Work out the finished part from the listing and answer in its coordinate system (mm). A direction names the side the tool comes from. Coordinates: 2 decimals unless noted, no trailing zeros. Order: outer loops, then holes, each group sorted by start corner. A loop starts at its lowest first (then second) coordinate and runs counter-clockwise, first axis right, second up. Notation, with made-up numbers: M 62.25,71 L 102.25,71 A21 cw 102.25,110 Z; hole C -25,3.5 d7. An arc over 180 degrees is marked long. Use a Markdown table: item, result.
Autodesk Inventor part; units mm, degrees
ref_plane "YZ Plane" through (0, 0, 0) normal (1, 0, 0) x (0, 1, 0)
ref_plane "XZ Plane" through (0, 0, 0) normal (0, 1, 0) x (-1, 0, 0)
ref_plane "XY Plane" through (0, 0, 0) normal (0, 0, 1) x (1, 0, 0)
sketch "Sketch1" plane through (0, 0, 0) normal (0, 1, 0) x (-1, 0, 0)
  line L0 (10.7, -12.7) -> (-10.7, -12.7)
  line L1 (-12.7, -10.7) -> (-12.7, 10.7)
  line L2 (-10.7, 12.7) -> (10.7, 12.7)
  line L3 (12.7, 10.7) -> (12.7, -10.7)
  line L4 (12.7, -10.7) -> (10.7, -12.7)
  line L5 (-10.7, -12.7) -> (-12.7, -10.7)
  line L6 (-12.7, 10.7) -> (-10.7, 12.7)
  line L7 (10.7, 12.7) -> (12.7, 10.7)
  circle A0 centre (9.525, -9.525) radius 1.27
  circle A1 centre (-9.525, 9.525) radius 1.27
  point P0 (0, 0)
  point P1 (12.7, -12.7)
  point P2 (-12.7, 12.7)
  point P3 (-12.7, -12.7)
  point P4 (12.7, 12.7)
  dimension "d0" = 25.4
  dimension "d2" = 25.4
  dimension "d3" = 12.7
  dimension "d4" = 12.7
  dimension "d5" = 2
  dimension "d6" = 2
  dimension "d7" = 2
  dimension "d8" = 2
  dimension "d9" = 2
  dimension "d10" = 2
  dimension "d11" = 2
  dimension "d12" = 2
  dimension "d13" = 3.175
  dimension "d14" = 3.175
  dimension "d15" = 3.175
  dimension "d16" = 3.175
  dimension "d17" = 2.54
  dimension "d18" = 2.54
extrude "Extrusion1" add sketch "Sketch1" along normal blind 26.9875
sketch "Sketch2" plane through (0, 26.9875, 0) normal (0, 1, 0) x (1, 0, 0)
  circle A0 centre (0, 0) radius 6.35
  circle A1 centre (0, 0) radius 3.175
  dimension "d21" = 12.7
  dimension "d23" = 6.35
extrude "Extrusion2" add sketch "Sketch2" along normal blind 2
sketch "Sketch3" plane through (0, 26.9875, 0) normal (0, 1, 0) x (1, 0, 0)
  circle A0 centre (0, 0) radius 6.35
  circle A1 centre (0, 0) radius 1.5
  dimension "d26" = 3
extrude "Extrusion3" add sketch "Sketch3" along normal blind 15 contours A1
sketch "Sketch4" plane through (0, 0, 0) normal (0, -1, 0) x (1, 0, 0)
  circle A0 centre (0, 0) radius 1.5
  dimension "d30" = 3
extrude "Extrusion4" add sketch "Sketch4" along normal blind 11.1125
sketch "Sketch5" plane through (0, 0, 0) normal (0, -1, 0) x (1, 0, 0)
  circle A0 centre (0, 0) radius 1.5
  circle A1 centre (0, 9.525) radius 0.7937
  circle A2 centre (9.525, 0) radius 0.7937
  line L0 (0, 0) -> (0, 9.525) construction
  line L1 (0, 0) -> (9.525, 0) construction
  dimension "d34" = 9.525
  dimension "d35" = 9.525
  dimension "d36" = 1.5875
  dimension "d37" = 1.5875
extrude "Extrusion5" add sketch "Sketch5" along normal blind 2.3813 contours A1 | A2
properties part number "launcher_motor"
1. Section D-D on x = 9.75 is taken. Determine the outline of the cut face in (y, z).
Answers below:
| item | result |
|---|---|
| outline | M -2.38,-0.76 L 0,-0.76 L 0,-12.7 L 26.99,-12.7 L 26.99,8.28 L 0,8.28 L 0,0.76 L -2.38,0.76 Z; M 0,10.77 L 26.99,10.77 L 26.99,12.7 L 0,12.7 Z |
2. Section A-A on y = 12 is taken. Determine the outline of the cut face in (x, z) (3 decimals).
Answers below:
| item | result |
|---|---|
| outline | M -12.7,-10.7 L -10.7,-12.7 L 10.7,-12.7 L 12.7,-10.7 L 12.7,10.7 L 10.7,12.7 L -10.7,12.7 L -12.7,10.7 Z; hole C -9.525,-9.525 d2.54; hole C 9.525,9.525 d2.54 |
3. For a pull along X with two mould halves and no side action, classify faces 5 (the face through (11.7, 13.3, -11.7)), 6 (the face through (-0.7, 26.988, 1.5)), 7 (the face through (-9.25, 13.305, -8.285)), 8 (the face through (-12.7, 13, 0)) as +X half, -X half, draft (parallel to the pull), parting line (faces both ways), or undercut.
Answers below:
| item | result |
|---|---|
| face 5 | +X half |
| face 6 | undercut |
| face 7 | undercut |
| face 8 | -X half |
4. Find the intervals of material crossed by probe 1 along Z at (x, y) = (0, 27.7) (3 decimals); probe 2 along X at (y, z) = (15.5, 9.5), in increasing order.
Answers below:
| item | result |
|---|---|
| probe 1 | -6.35 to -3.175, -1.5 to 1.5, 3.175 to 6.35 |
| probe 2 | -12.7 to 8.26, 10.79 to 12.7 |
5. Flat-ended cylindrical pins translate along their axes: P1, Ø1, axis at x = -0.5, y = 35, coming from the -Z side; P2, Ø1.7, axis at x = 9.5, z = 0.5, coming from the -Y side; P3, Ø10, axis at x = 8, z = -3, coming from the +Y side; P4, Ø2, axis at x = -9.525, z = -9.525, coming from the +Y side. Find the tip coordinate at first contact, or state that the pin passes through.
Answers below:
| item | result |
|---|---|
| P1 | z = -1.5 |
| P2 | y = -2.38 |
| P3 | y = 28.99 |
| P4 | through |
6. For faces 1 (the face through (10.28, -1.17, -0.24)), 2 (the face through (0, -2.381, 10)), 3 (the face through (10, -2.381, 0)), 4 (the face through (-0.69, 27.97, -3.1)), determine the directions among +Z, -Z, +X, -X, +Y, -Y from which every point of the face is accessible in a straight line to the end or side of a thin tool.
Answers below:
| item | result |
|---|---|
| face 1 | -Y |
| face 2 | +Z, +X, -X, -Y |
| face 3 | +Z, -Z, +X, -Y |
| face 4 | +Y |
